Input: part model. Units: mm. Frame: model coordinates. Face numbers are marked on the shaded views. A direction names the side the tool comes from. Give positions to 0.01 mm unless a question says otherwise; leave off trailing zeros. Loops run counter-clockwise (first coordinate to the right, second up) from the corner with the lowest first, then second, coordinate; pieces in that order, holes last. Notation, with made-up numbers: (-24, 14.25) - (13, 14.25) arc R29 cw to (13, 39.25) - close; hole circle Ø6 at (63, 28). An arc over 180 degrees is marked (long way). Answer as a JSON object with one key per item and string values. Group by question number.
(1) Material intervals for L1, parallel to Z at x = -12, y = 1.85; L2, parallel to X at y = 1.2, z = -12; L3, parallel to X at y = 2.6, z = 0, sorted ascending.
(2) Pin query (flat end, axial travel): P1, Ø0.8, axis at x = -9.5, y = 5.5, coming from the -Z side; P2, Ø3, axis at x = -5.5, z = 17.5, coming from the +Y side; P3, Ø0.5, axis at x = 0, y = 5.5, coming from the -Z side. Return the tip coordinate at first contact, or that it passes through.
(3) Section query D-D (x = 23). Return loops of the section in (y, z), plus the area to 3 significant figures.
(4) Section query C-C (z = -9.5). Return loops of the section in (x, y).
(5) Section query B-B (x = -8). Return loops of the section in (y, z).
(6) Access query for the marked faces 1, 2 and 3. Directions: +Z, -Z, +X, -X, +Y, -Y. A direction counts if a zero-diameter tool reaches every point of the face in a straight line with its end or side. Return the directions, or none.
(7) Section query A-A (y = 1.15). Count the separate pieces of the cut face and the enclosed holes in it, plus the area to 3 significant figures.
```python
from build123d import *

# Parameters (mm, degrees)
BOSS_EXTRU_1_DEPTH      = 5
BOSS_EXTRU_2_DEPTH      = 1
ESQUISSE3_W             = 5.2
ESQUISSE3_H             = 5.2
ESQUISSE3_W_2           = 5
ESQUISSE3_H_2           = 5
ENL_V_MAT_EXTRU_1_DEPTH = 4.8
CONG_1_R                = 10
CONG_2_R                = 5


with BuildPart() as part:
    # Esquisse1 → Boss.-Extru.1 (new body)
    with BuildSketch(Plane(origin=(0, 0, 0), x_dir=(1, 0, 0), z_dir=(0, 1, 0))):
        Polygon((22, 13), (12.003020456, 23), (-12.003020456, 23), (-22, 13), (-22, -13), (-12.003020456, -23), (12.003020456, -23), (22, -13), (22, -5), (26, -5), (26, 5), (22, 5), align=None)
    extrude(amount=BOSS_EXTRU_1_DEPTH)

    # Esquisse2 → Boss.-Extru.2 (add)
    with BuildSketch(Plane(origin=(0, 5, 0), x_dir=(1, 0, 0), z_dir=(0, 1, 0))):
        Polygon((-12.651968736, 13), (-12.651968736, 8), (3.556100985, 8), (3.556100985, -2), (-2.443899015, -2), (6.056100985, -15.555441712), (14.556100985, -2), (8.556100985, -2), (8.556100985, 13), align=None)
    extrude(amount=BOSS_EXTRU_2_DEPTH)

    # Esquisse3 → Enlèv. mat.-Extru.1 (cut)
    with BuildSketch(Plane.XZ):
        with Locations((-13.4, 14.4)):
            Rectangle(ESQUISSE3_W, ESQUISSE3_H)
        with Locations((-13.4, -14.4)):
            Rectangle(ESQUISSE3_W, ESQUISSE3_H)
        with Locations((14.4, -14.4)):
            Rectangle(ESQUISSE3_W, ESQUISSE3_H)
        with Locations((13.4, 14.4)):
            Rectangle(ESQUISSE3_W, ESQUISSE3_H)
        Rectangle(ESQUISSE3_W_2, ESQUISSE3_H_2)
    extrude(amount=-ENL_V_MAT_EXTRU_1_DEPTH, mode=Mode.SUBTRACT)

    # Congé1
    cong_1_edges = [part.edges().sort_by_distance(p)[0] for p in [
        (8.556100985, 5.5, -13),
    ]]
    fillet(cong_1_edges, radius=CONG_1_R)

    # Congé2
    cong_2_edges = [part.edges().sort_by_distance(p)[0] for p in [
        (3.556100985, 5.5, -8),
    ]]
    fillet(cong_2_edges, radius=CONG_2_R)


solid = part.part
```
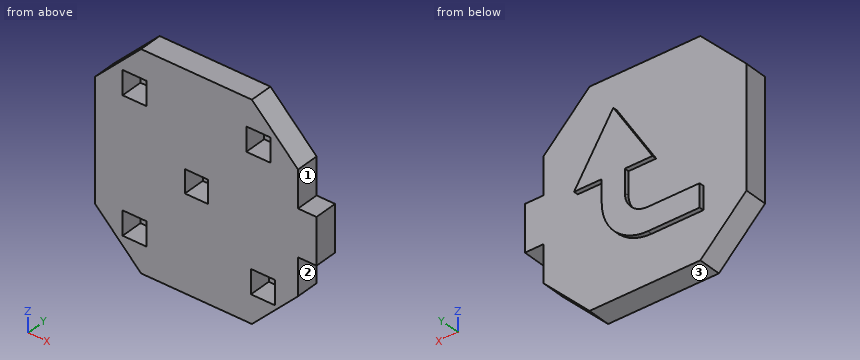
Recorded:
{
 "1": {"L1": "z = -23 to -17, -11.8 to 11.8, 17 to 23", "L2": "x = -22 to -16, -10.8 to 11.8, 17 to 22", "L3": "x = -22 to -2.5, 2.5 to 26"},
 "2": {"P1": "stops at z = -13", "P2": "stops at y = 5", "P3": "stops at z = -12.93"},
 "3": {"outline": "(0, -5) - (5, -5) - (5, 5) - (0, 5) - close", "area": "50.0 mm^2"},
 "4": {"outline": "(-22, 0) - (22, 0) - (22, 5) - (6.16, 5) - (6.16, 6) - (-12.65, 6) - (-12.65, 5) - (-22, 5) - close"},
 "5": {"outline": "(0, -23) - (5, -23) - (5, -13) - (6, -13) - (6, -8) - (5, -8) - (5, 23) - (0, 23) - close"},
 "6": {"face 1": "+Z, +X, +Y, -Y", "face 2": "-Z, +X, +Y, -Y", "face 3": "-Z, +X, -X, +Y, -Y"},
 "7": {"separate pieces": "1", "enclosed holes": "5", "area": "1,730 mm^2"}
}
